```python
from build123d import *

# Parameters (mm, degrees)
F0_W     = 895.35
F0_H     = 533.4
F0_W_2   = 882.65
F0_H_2   = 520.7
F1_DEPTH = 76.2
F2_DEPTH = 3.175
F3_W     = 6.35
F3_H     = 82.55
F4_DEPTH = 76.2
F5_W     = 146.05
F5_H     = 63.5
F6_DEPTH = 895.351


with BuildPart() as f1:
    # F0 (on Top) → F1 (new body)
    with BuildSketch(Plane.XY):
        Rectangle(F0_W, F0_H)
        Rectangle(F0_W_2, F0_H_2, mode=Mode.SUBTRACT)
    extrude(amount=F1_DEPTH)

    # F0 (on Top) → F2 (join)
    with BuildSketch(Plane.XY):
        Rectangle(F0_W_2, F0_H_2)
    extrude(amount=F2_DEPTH)

    # F3 (on face) → F4 (join)
    with BuildSketch(Plane.XY.offset(76.2)):
        with Locations((-444.5, -41.275)):
            Rectangle(F3_W, F3_H)
        with Locations((-444.5, 41.275)):
            Rectangle(F3_W, F3_H)
        with Locations((444.5, 41.275)):
            Rectangle(F3_W, F3_H)
        with Locations((444.5, -41.275)):
            Rectangle(F3_W, F3_H)
    extrude(amount=F4_DEPTH)

    # F5 (on face) → F6 (cut, through all)
    with BuildSketch(Plane(origin=(-447.675, 0, 0), x_dir=(0, -1, 0), z_dir=(-1, 0, 0))):
        with Locations((0, 107.95)):
            Rectangle(F5_W, F5_H)
    extrude(amount=-F6_DEPTH, mode=Mode.SUBTRACT)


solid = f1.part
```
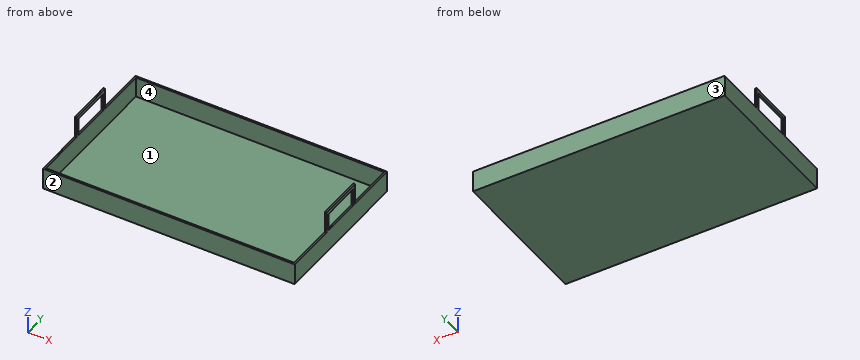
Read the model definition and answer for the solid it produces. Units are mm, in the model's axes. Face numbers are marked on the shaded views. A direction names the side the tool comes from. Give positions to 0.01 mm unless a question says otherwise; leave off trailing zeros. Write each loop counter-clockwise with the first axis right and the second up, starting at its lowest first coordinate (ties: lowest second). Pieces come first, ordered by that corner, then holes. Notation, with made-up numbers: (-3.75, -26) -> (53.25, -26) arc R29 ccw to (53.25, -4) -> close; hole circle Ø2 at (33.5, 79). An arc over 180 degrees is marked (long way). Answer in a Markdown table with one row per item.
1) Determine the mould class of the marked faces 1 and 2 for opening direction X: released by +X, released by -X, zero draft, split by the parting line, or undercut.
Results list:
| item | result |
|---|---|
| face 1 | undercut |
| face 2 | zero draft |
2) Straight lines are drawn through the part: line 1 (Y direction, x = -347.5, z = 8.5); line 2 (X direction, y = -102.5, z = 22) (3 decimals); line 3 (Z direction, x = 353.5, y = 105) (3 decimals). For each, find the intervals that lie inside material, in ascending order. Write a range as [from, to].
Results list:
| item | result |
|---|---|
| line 1 | [-266.7, -260.35], [260.35, 266.7] |
| line 2 | [-447.675, -441.325], [441.325, 447.675] |
| line 3 | [0, 3.175] |
3) Each of these flat-tipped pins is pushed along its axis until it touches: pin 1 Ø8 at (x, y) = (182, -112) entering from -Z; pin 2 Ø7 at (x, z) = (-443, 125) entering from +Y; pin 3 Ø3 at (x, z) = (445, 96) entering from -Y; pin 4 Ø1.5 at (y, z) = (-147.5, 77) entering from +X. Where does it stop, or does it pass through?
Results list:
| item | result |
|---|---|
| pin 1 | z = 0 |
| pin 2 | y = 82.55 |
| pin 3 | y = -82.55 |
| pin 4 | through |
4) A tool of negligible diameter and unlimited length cuts with its end or side. For the marked faces 3 and 4, from which of +Z, -Z, +X, -X, +Y, -Y can it reach the whole face along a straight path? Write none if from no direction.
Results list:
| item | result |
|---|---|
| face 3 | +Z, -Z, +X, -X, +Y |
| face 4 | +Z |
5) Section A-A on z = 127.5 is taken. Give the vertices of the cut face in (x, y) (3 decimals), plus the area to 3 significant figures.
Results list:
| item | result |
|---|---|
| outline | (-447.675, -82.55) -> (-441.325, -82.55) -> (-441.325, -73.025) -> (-447.675, -73.025) -> close; (-447.675, 73.025) -> (-441.325, 73.025) -> (-441.325, 82.55) -> (-447.675, 82.55) -> close; (441.325, -82.55) -> (447.675, -82.55) -> (447.675, -73.025) -> (441.325, -73.025) -> close; (441.325, 73.025) -> (447.675, 73.025) -> (447.675, 82.55) -> (441.325, 82.55) -> close |
| area | 242 mm^2 |
6) Section C-C on x = -116 is taken. Give the vertices of the cut face in (y, z) (3 decimals).
Results list:
| item | result |
|---|---|
| outline | (-266.7, 0) -> (266.7, 0) -> (266.7, 76.2) -> (260.35, 76.2) -> (260.35, 3.175) -> (-260.35, 3.175) -> (-260.35, 76.2) -> (-266.7, 76.2) -> close |
7) Section D-D on y = 94 is taken. Give the vertices of the cut face in (x, z) (3 decimals), plus the area to 3 significant figures.
Results list:
| item | result |
|---|---|
| outline | (-447.675, 0) -> (447.675, 0) -> (447.675, 76.2) -> (441.325, 76.2) -> (441.325, 3.175) -> (-441.325, 3.175) -> (-441.325, 76.2) -> (-447.675, 76.2) -> close |
| area | 3,770 mm^2 |
8) Section B-B on y = -15 is taken. Give the vertices of the cut face in (x, z) (3 decimals), plus the area to 3 significant figures.
Results list:
| item | result |
|---|---|
| outline | (-447.675, 0) -> (447.675, 0) -> (447.675, 76.2) -> (441.325, 76.2) -> (441.325, 3.175) -> (-441.325, 3.175) -> (-441.325, 76.2) -> (-447.675, 76.2) -> close; (-447.675, 139.7) -> (-441.325, 139.7) -> (-441.325, 152.4) -> (-447.675, 152.4) -> close; (441.325, 139.7) -> (447.675, 139.7) -> (447.675, 152.4) -> (441.325, 152.4) -> close |
| area | 3,930 mm^2 |
